Geometry: final body of the model. Coordinates: model frame, mm. A direction names the side the tool comes from. Give positions to 0.01 mm unless a question says otherwise; leave off trailing zeros. Order: outer loops, then holes, each group sorted by start corner. A loop starts at its lowest first (then second) coordinate and runs counter-clockwise, first axis right, second up. Notation, with made-up numbers: (34.25, 52) - (87.25, 52) arc R23 ccw to (87.25, 90) - close; hole circle Ø3 at (49.5, -0.75). An arc over 180 degrees is marked (long way). Put each result on its own line as item: value. Start each with the question number.
1. Section B-B on z = -23. Return the cut outline in (x, y).
2. Ray query, line 1 along Z through (x, y) = (-4.6, 1.6); line 2 along X through (y, z) = (1.75, -4); line 3 along X through (y, z) = (14, -60). Return the intervals inside material, ascending. Write a range as from..to.
3. Mould query, pull axis Z, two halves, no side actions, for faces 4 (the flat face through (10.25, 5, -16)), 5 (the flat face through (13.493, 5, -26)), 6 (the flat face through (-29.383, 4.055, -46.311)). Classes: pulls with the +Z half, pulls with the -Z half, needs draft (parallel to the pull), parting line crosses it, or undercut.
4. Set-up query: faces 1 (the flat face through (0, 2, 30)), 2 (the flat face through (17, 2.5, -26)), 3 (the flat face through (0, 2.5, 22)). Return all of +Z, -Z, +X, -X, +Y, -Y with unobstructed straight access to the full face (end or side cutting, diameter ignored); none if empty.
5. Section A-A on y = 15. Return the cut outline in (x, z).
6. Section C-C on x = -4.8. Count the separate pieces of the cut face and the enclosed holes in it, plus the area to 3 significant figures.
7. First-contact query: P1, Ø4, axis at y = 3.5, z = -3.5, coming from the -X side; P2, Ø7.5, axis at x = -4.8, z = -30.31, coming from the +Y side; P3, Ø4, axis at y = 9.5, z = -61.5, coming from the +X side. Flat tips, straight axial feed; report the tip coordinate or a pass-through.
from build123d import *

# Parameters (mm, degrees)
BOSS_EXTRUDE1_DEPTH      = 2.5
SKETCH2_W                = 20.5
SKETCH2_H                = 41.5
CUT_EXTRUDE1_DEPTH       = 3.5
SKETCH8_R                = 2.3
CUT_EXTRUDE2_DEPTH       = 3.5
BOSS_EXTRUDE2_DEPTH      = 10
BOSS_EXTRUDE2_TAPER      = 15
SKETCH10_R               = 7.5
BOSS_EXTRUDE3_DEPTH      = 20
BOSS_EXTRUDE3_DEPTH_BACK = 2.5
SKETCH11_R               = 2
CUT_EXTRUDE3_DEPTH       = 23.5
BOSS_EXTRUDE7_DEPTH      = 10
CUT_EXTRUDE4_DEPTH       = 42
CUT_EXTRUDE4_DEPTH_BACK  = 42


with BuildPart() as part:
    # Sketch1 → Boss-Extrude1 (new body)
    with BuildSketch(Plane(origin=(0, 0, 0), x_dir=(1, 0, 0), z_dir=(0, 1, 0))):
        Polygon((-25, 30), (-32.256053395, 57), (-47.256053395, 57), (-66, 52), (-66, 62), (-50, 72), (-32.256053395, 80), (32.256053395, 80), (50, 72), (66, 62), (66, 52), (47.256053395, 57), (32.256053395, 57), (25, 30), (25, -30), (-25, -30), align=None)
    extrude(amount=BOSS_EXTRUDE1_DEPTH)

    # Sketch2 → Cut-Extrude1 (cut, through all)
    with BuildSketch(Plane(origin=(0, 2.5, 0), x_dir=(1, 0, 0), z_dir=(0, 1, 0))):
        with Locations((0, 5.559891181)):
            Rectangle(SKETCH2_W, SKETCH2_H)
    extrude(amount=-CUT_EXTRUDE1_DEPTH, mode=Mode.SUBTRACT)

    # Sketch8 → Cut-Extrude2 (cut, through all)
    with BuildSketch(Plane(origin=(0, 2.5, 0), x_dir=(1, 0, 0), z_dir=(0, 1, 0))):
        with Locations((-4.8, 30.309891181)):
            Circle(SKETCH8_R)
        with Locations((4.8, 30.309891181)):
            Circle(SKETCH8_R)
        with Locations((-4.6, -19.190108819)):
            Circle(SKETCH8_R)
        with Locations((4.6, -19.190108819)):
            Circle(SKETCH8_R)
    extrude(amount=-CUT_EXTRUDE2_DEPTH, mode=Mode.SUBTRACT)

    # Sketch9 → Boss-Extrude2 (add)
    with BuildSketch(Plane(origin=(0, 2.5, 0), x_dir=(1, 0, 0), z_dir=(0, 1, 0))):
        Polygon((-65, 62.845048963), (-65, 55), (-50, 58), (-35.31985343, 60), (35.31985343, 60), (50, 58), (65, 55), (65, 62.845048963), (50, 68), (35.31985343, 70), (-35.31985343, 70), (-50, 68), align=None)
    extrude(amount=BOSS_EXTRUDE2_DEPTH, taper=BOSS_EXTRUDE2_TAPER)

    # Sketch10 → Boss-Extrude3 (add, two sides)
    with BuildSketch(Plane(origin=(0, 2.5, 0), x_dir=(1, 0, 0), z_dir=(0, 1, 0))) as boss_extrude3_sk:
        with Locations((-62.320508076, 58.268454707)):
            Circle(SKETCH10_R)
        with Locations((62.320508076, 58.268454707)):
            Circle(SKETCH10_R)
    extrude(amount=BOSS_EXTRUDE3_DEPTH)
    extrude(boss_extrude3_sk.sketch, amount=-BOSS_EXTRUDE3_DEPTH_BACK)

    # Sketch11 → Cut-Extrude3 (cut, through all)
    with BuildSketch(Plane(origin=(0, 22.5, 0), x_dir=(1, 0, 0), z_dir=(0, 1, 0))):
        with Locations((-62.320508076, 58.268454707)):
            Circle(SKETCH11_R)
        with Locations((62.320508076, 58.268454707)):
            Circle(SKETCH11_R)
    extrude(amount=-CUT_EXTRUDE3_DEPTH, mode=Mode.SUBTRACT)

    # Sketch12 → Boss-Extrude7 (add)
    with BuildSketch(Plane(origin=(0, 2.5, 0), x_dir=(1, 0, 0), z_dir=(0, 1, 0))):
        Polygon((-25, -30), (-25, 30), (-32.256053395, 57), (-32.256053395, 65.259387318), (-27.256053395, 65.259387318), (-27.256053395, 57.660145211), (-20, 30.660145211), (-20, -30), align=None)
        Polygon((-10.25, -15.190108819), (-10.25, -30), (-13.493333109, -30), (-13.493333109, 64.72993517), (-10.25, 64.72993517), (-10.25, 26.309891181), align=None)
    boss_extrude7 = extrude(amount=BOSS_EXTRUDE7_DEPTH)

    # Mirror2: Boss-Extrude7 across plane
    add(boss_extrude7.mirror(Plane(origin=(0, 0, 0), x_dir=(0, 0, 1), z_dir=(1, 0, 0))))

    # Sketch13 → Cut-Extrude4 (cut, two sides)
    with BuildSketch(Plane(origin=(0, 0, 0), x_dir=(0, 0, -1), z_dir=(1, 0, 0))) as cut_extrude4_sk:
        Polygon((-30, 6.091325502), (41.254032245, 6.091325502), (62.608757253, 12.229145442), (-30, 17.289989114), align=None)
    extrude(amount=CUT_EXTRUDE4_DEPTH, mode=Mode.SUBTRACT)
    extrude(cut_extrude4_sk.sketch, amount=-CUT_EXTRUDE4_DEPTH_BACK, mode=Mode.SUBTRACT)


solid = part.part
Resolved:
1. outline: (-25, 0) - (-10.25, 0) - (-10.25, 6.09) - (-13.49, 6.09) - (-13.49, 2.5) - (-20, 2.5) - (-20, 6.09) - (-25, 6.09) - close; (10.25, 0) - (25, 0) - (25, 6.09) - (20, 6.09) - (20, 2.5) - (13.49, 2.5) - (13.49, 6.09) - (10.25, 6.09) - close
2. line 1: -80..-32.6, -28.02..-26.31, 15.19..16.89, 21.49..30
2. line 2: -25..-10.25, 10.25..25
2. line 3: -69.62..-63.32, -61.32..-55.02, 55.02..61.32, 63.32..69.62
3. face 4: undercut
3. face 5: needs draft
3. face 6: pulls with the +Z half
4. face 1: +Z, +X, -X, +Y, -Y
4. face 2: +Y
4. face 3: +Z, +Y
5. outline: circle Ø15 at (-62.32, -58.27); circle Ø15 at (62.32, -58.27); hole circle Ø4 at (-62.32, -58.27); hole circle Ø4 at (62.32, -58.27)
6. separate pieces: 4
6. enclosed holes: 0
6. area: 221 mm^2
7. P1: x = -25
7. P2: y = 2.5
7. P3: x = 69.72
